Autodesk Inventor part; units mm, degrees
ref_plane "YZ Plane" through (0, 0, 0) normal (1, 0, 0) x (0, 1, 0)
ref_plane "XZ Plane" through (0, 0, 0) normal (0, 1, 0) x (-1, 0, 0)
ref_plane "XY Plane" through (0, 0, 0) normal (0, 0, 1) x (1, 0, 0)
sketch "スケッチ1" plane through (0, 0, 0) normal (0, 0, 1) x (1, 0, 0)
  arc A0 (-81.314, -122.2088) -> (79.2809, -122.2088) centre (-1.0165, 49.9897) ccw
  line L0 (-1.0165, 49.9897) -> (79.2809, -122.2088) construction
  line L1 (-1.0165, 49.9897) -> (188.9835, 49.9897) construction
  line L2 (-1.0165, 49.9897) -> (-81.314, -122.2088) construction
  arc A1 (-79.2009, -117.6773) -> (77.1678, -117.6773) centre (-1.0165, 49.9897) ccw
  line L3 (-1.0165, 49.9897) -> (77.1678, -117.6773) construction
  line L4 (-1.0165, 49.9897) -> (183.9835, 49.9897) construction
  line L5 (-1.0165, 49.9897) -> (-79.2009, -117.6773) construction
  line L6 (0, -135.0075) -> (35, -74.3858)
  line L7 (0, -135.0075) -> (70, -135.0075) construction
  line L8 (35, -74.3858) -> (2.1456, -4.5601)
  line L9 (35, -74.3858) -> (112.1689, -74.3858) construction
  circle A2 centre (0, 0) radius 2
  circle A3 centre (0, 0) radius 3.075
  circle A4 centre (0, 0) radius 6.5
  line L10 (0, 0) -> (33.3477, -70.8742) construction
  line L11 (-4.5242, -2.1287) -> (28.8235, -73.0029)
  line L12 (37.8719, -68.7455) -> (4.5242, 2.1287)
  arc A5 (4.5242, 2.1287) -> (-4.5242, -2.1287) centre (0, 0) ccw
  arc A6 (28.8235, -73.0029) -> (37.8719, -68.7455) centre (33.3477, -70.8742) ccw
  line L13 (-1.0165, -135.0103) -> (33.3477, -70.8742) construction
  line L14 (3.3907, -137.3717) -> (37.755, -73.2356)
  line L15 (28.9405, -68.5128) -> (-5.4238, -132.6489)
  arc A7 (-5.4238, -132.6489) -> (3.3907, -137.3717) centre (-1.0165, -135.0103) ccw
  arc A8 (37.755, -73.2356) -> (28.9405, -68.5128) centre (33.3477, -70.8742) ccw
  arc A9 (-80.0461, -119.4899) -> (78.0131, -119.4899) centre (-1.0165, 49.9897) ccw
  line L16 (-1.0165, 49.9897) -> (78.0131, -119.4899) construction
  line L17 (-1.0165, 49.9897) -> (185.9835, 49.9897) construction
  line L18 (-1.0165, 49.9897) -> (-80.0461, -119.4899) construction
  line L19 (0, 0) -> (19.103, -135.9248)
  line L20 (0, 0) -> (137.2607, 0) construction
  line L21 (33.3477, -70.8742) -> (19.103, -135.9248) construction
  line L22 (28.4635, -69.8046) -> (14.2187, -134.8553)
  line L23 (23.9873, -136.9944) -> (38.232, -71.9437)
  arc A10 (38.232, -71.9437) -> (28.4635, -69.8046) centre (33.3477, -70.8742) ccw
  arc A11 (14.2187, -134.8553) -> (23.9873, -136.9944) centre (19.103, -135.9248) ccw
  point P0 (0, 0)
  point P1 (16.6739, -35.4371)
  point P2 (16.1656, -102.9423)
  point P3 (6.2925, -1.6294)
  point P4 (-2.756, -5.8868)
  point P5 (27.7533, -70.7285)
  point P6 (37.8719, -68.7455)
  point P7 (-5.6235, -136.9536)
  point P8 (3.6151, -136.953)
  point P9 (37.755, -73.2356)
  point P10 (37.8719, -68.7455)
  point P11 (33.3512, -133.8251)
  point P12 (26.2254, -103.3995)
  point P13 (28.0999, -71.465)
  point P14 (14.1253, -136.3963)
  point P15 (24.3626, -135.2801)
  dimension "d0" = 50
  dimension "d1" = 190
  dimension "d2" = 65
  dimension "d3" = 50
  dimension "d4" = 185
  dimension "d5" = 65
  dimension "d6" = 50
  dimension "d7" = 70
  dimension "d8" = 60
  dimension "d9" = 0
  dimension "d11" = 4
  dimension "d12" = 6.15
  dimension "d13" = 13
  dimension "d14" = 10
  dimension "d15" = 10
  dimension "d16" = 187
  dimension "d17" = 65
  dimension "d18" = 50
  dimension "d34" = 0
  dimension "d35" = 0
  dimension "d36" = 82
  dimension "d37" = 10
extrude "押し出し1" add sketch "スケッチ1" along normal mid plane 5 contours A3
extrude "押し出し2" add sketch "スケッチ1" along normal mid plane 10 contours L11 L19 A4 L8 A8 L15 | L11 A4 L19 | L11 A5 L12 A4 | A4 L12 A5 L11 | A8 L8 A4 L12
extrude "押し出し3" add sketch "スケッチ1" along normal mid plane 10 contours A11 L22 A1 L19 A9 | L19 A1 L23 A9 | L19 L22 L14 A6 L23 A1 | A1 L22 L19 | L22 L11 A6 L6 | L6 A6 L14 L22 | L15 A10 L22 L11 | A6 L6 L8 A8 | A6 L11 L22 A10 A8 L8 L6
sketch "スケッチ2" plane through (0, 0, 5) normal (0, 0, 1) x (1, 0, 0)
  line L0 (-17.1369, -20) -> (12.9571, -20)
  arc A0 (-63.3927, -125.9462) -> (63.3927, -125.9462) centre (0, 10) ccw
  line L1 (0, 10) -> (63.3927, -125.9462) construction
  line L2 (0, 10) -> (150, 10) construction
  line L3 (0, 10) -> (-63.3927, -125.9462) construction
  arc A1 (-61.2796, -121.4146) -> (61.2796, -121.4146) centre (0, 10) ccw
  line L4 (0, 10) -> (61.2796, -121.4146) construction
  line L5 (0, 10) -> (145, 10) construction
  line L6 (0, 10) -> (-61.2796, -121.4146) construction
  line L7 (-63.3927, -125.9462) -> (-61.2796, -121.4146)
  line L8 (63.3927, -125.9462) -> (61.2796, -121.4146)
  point P0 (0, 0)
  point P1 (0, -20)
  dimension "d25" = 20
  dimension "d26" = 10
  dimension "d27" = 150
  dimension "d28" = 65
  dimension "d29" = 50
  dimension "d30" = 145
  dimension "d31" = 65
  dimension "d32" = 50
revolve "回転1" add sketch "スケッチ2" angle 35 about axis through (-17.1369, -20, 5) along (1, 0, 0)
sketch "スケッチ3" plane through (0, 0, 0) normal (0, 1, 0) x (-1, 0, 0)
  line L0 (-14.3428, 5) -> (61.2796, 5)
  circle A0 centre (20, -2) radius 2.5
  line L1 (20, 3) -> (24.3301, 0.5)
  line L2 (24.3301, 0.5) -> (24.3301, -4.5)
  line L3 (24.3301, -4.5) -> (20, -7)
  line L4 (20, -7) -> (15.6699, -4.5)
  line L5 (15.6699, -4.5) -> (15.6699, 0.5)
  line L6 (15.6699, 0.5) -> (20, 3)
  circle A1 centre (40, -2) radius 2.5
  line L7 (40, 3) -> (35.6699, 0.5)
  line L8 (35.6699, 0.5) -> (35.6699, -4.5)
  line L9 (35.6699, -4.5) -> (40, -7)
  line L10 (40, -7) -> (44.3301, -4.5)
  line L11 (44.3301, -4.5) -> (44.3301, 0.5)
  line L12 (44.3301, 0.5) -> (40, 3)
  point P0 (0, 0)
  dimension "d38" = 7
  dimension "d39" = 20
  dimension "d40" = 5
  dimension "d41" = 10
extrude "押し出し4" cut sketch "スケッチ3" against normal blind 1000 contours A0 | A1
extrude "押し出し5" cut sketch "スケッチ3" against normal blind 132 contours L12 L11 L10 L9 L8 L7
extrude "押し出し6" cut sketch "スケッチ3" against normal blind 137 contours L1 L2 L3 L4 L5 L6
properties part number "passive_walking_robot5"
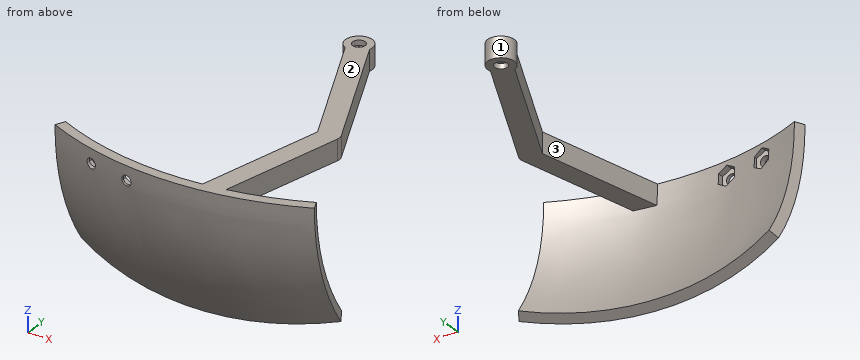
Model file for the job. Use its own axes, mm. Face numbers are marked on the shaded views. Give positions to 0.01 mm unless a question says otherwise; leave off trailing zeros. Loops run counter-clockwise (first coordinate to the right, second up) from the corner with the lowest first, then second, coordinate; pieces in that order, holes last.
1) Wall check: line 1 (Y direction, x = 0, z = -3.35) (3 decimals); line 2 (Y direction, x = -30, z = -41.5); line 3 (Z direction, x = -40, y = -134.4). Give the ranges that are in metal, low to high.
2) Pull direction X, two halves, no side cores. Call the marked faces 1, 2 and 3: +X half, -X half, draft (parallel to the pull), parting line (faces both ways), or undercut.
3) Flat gauge pins, fed straight in: pin 1 Ø1.5 at (x, z) = (-10, -47.5) entering from +Y; pin 2 Ø1.8 at (x, y) = (1.5, 0) entering from +Z; pin 3 Ø4.5 at (x, z) = (-40, -4.5) entering from +Y. Where does each tip first touch, or does it go through?
4) Saw through at B-B (y = -20). Write the cut outline in (x, z), plus the area to 3 significant figures.
5) Saw through at A-A (x = 0). Count the separate pieces of the cut face and the enclosed holes in it, plus the area to 3 significant figures.
6) Saw through at C-C (y = -89.5). Write the cut outline in (x, z).
Answer block:
1. line 1: y = -139.709 to -134.696, -11.744 to -3.075, 3.075 to 6.5
1. line 2: y = -127.33 to -121.74
1. line 3: z = 0.5 to 5
2. face 1: parting line
2. face 2: draft
2. face 3: undercut
3. pin 1: stops at y = -121.53
3. pin 2: stops at z = 2.5
3. pin 3: stops at y = -128.34
4. outline: (3.88, -5) - (14.94, -5) - (14.94, 5) - (3.88, 5) - close
4. area: 111 mm2
5. separate pieces: 3
5. enclosed holes: 0
5. area: 491 mm2
6. outline: (24.15, -5) - (34.39, -5) - (34.39, 5) - (24.15, 5) - close
